```python
from build123d import *

# Parameters (mm, degrees)
SKETCH1_W           = 25.6
SKETCH1_H           = 25.6
BOSS_EXTRUDE1_DEPTH = 15.24
SKETCH2_R           = 2.5
CUT_EXTRUDE1_DEPTH  = 33.426186948
SKETCH3_R           = 1.25
CUT_EXTRUDE2_DEPTH  = 24.663000655
CHAMFER1_SIZE       = 0.5
SKETCH7_R           = 3
CUT_EXTRUDE3_DEPTH  = 24.663000655


with BuildPart() as part:
    # Sketch1 → Boss-Extrude1 (new body)
    with BuildSketch(Plane(origin=(0, 0, 0), x_dir=(1, 0, 0), z_dir=(0, 1, 0))):
        Rectangle(SKETCH1_W, SKETCH1_H)
    extrude(amount=BOSS_EXTRUDE1_DEPTH)

    # Sketch2 → Cut-Extrude1 (cut, through all)
    with BuildSketch(Plane.XY.offset(12.8)):
        with Locations((-8.05, 6.74)):
            Circle(SKETCH2_R)
        with Locations((8.05, 6.74)):
            Circle(SKETCH2_R)
    extrude(amount=-CUT_EXTRUDE1_DEPTH, mode=Mode.SUBTRACT)

    # Sketch3 → Cut-Extrude2 (cut, through all)
    with BuildSketch(Plane(origin=(0, 15.24, 0), x_dir=(1, 0, 0), z_dir=(0, 1, 0))):
        with Locations(Location((0, -8.3, 0), (0, 0, 270))):
            Circle(SKETCH3_R)
    extrude(amount=-CUT_EXTRUDE2_DEPTH, mode=Mode.SUBTRACT)

    # Chamfer1
    chamfer1_edges = [part.edges().sort_by_distance(p)[0] for p in [
        (-10.55, 6.74, -12.8),
        (-10.55, 6.74, 12.8),
        (5.55, 6.74, -12.8),
        (5.55, 6.74, 12.8),
        (0, 0, 7.05),
        (0, 15.24, 7.05),
    ]]
    chamfer(chamfer1_edges, length=CHAMFER1_SIZE)

    # Sketch7 → Cut-Extrude3 (cut, through all)
    with BuildSketch(Plane(origin=(0, 15.24, 0), x_dir=(1, 0, 0), z_dir=(0, 1, 0))):
        with Locations(Location((0, 0, 0), (0, 0, 270))):
            Circle(SKETCH7_R)
    extrude(amount=-CUT_EXTRUDE3_DEPTH, mode=Mode.SUBTRACT)


solid = part.part
```
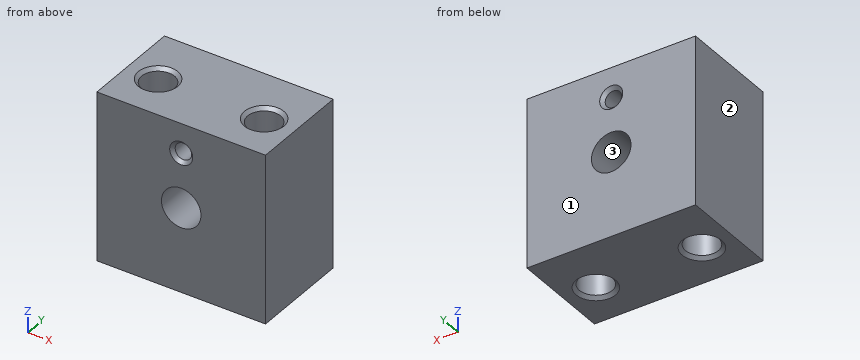
For this review, take the finished solid that the model builds, in its own axes (mm). Face numbers are marked on the shaded views. Give positions to 0.01 mm unless a question says otherwise; leave off trailing zeros. Order: outer loops, then holes, each group sorted by start corner. A loop starts at its lowest first (then second) coordinate and runs counter-clockwise, first axis right, second up.
1) Insertion check: pin 1 (3 mm diameter, centred on x = 0, z = 8.3, fed in from -Y). The pin has a flat end and moves straight along its axis. Give the tip position at first contact, or say it passes through.
2) Wall thickness on line 1 (X direction, y = 8.75, z = 6.5); line 2 (X direction, y = 4.75, z = 7.5); line 3 (Y direction, x = 8.05, z = -2.5): over which ranges is each line inside the solid? List them lowest first.
3) Take a section at B-B (z = 0). Give the boundary of the cut face in (x, y).
4) Take a section at A-A (y = 6.74). Give the boundary of the cut face in (x, z).
5) The part is to be moulded in two halves that separate along X. For the marked faces 1, 2 and 3, say which applies: released by +X, released by -X, zero draft, split by the parting line, or undercut.
6) Take a section at C-C (x = 8.05). Give the boundary of the cut face in (y, z), then the cut area to 3 significant figures.
7) Take a section at D-D (z = -3.5). Give the boundary of the cut face in (x, y), then the cut area to 3 significant figures.
Derived:
1. pin 1: stops at y = 0.25
2. line 1: x = -12.8 to -9.54, -6.56 to 6.56, 9.54 to 12.8
2. line 2: x = -12.8 to -9.56, -6.54 to -0.96, 0.96 to 6.54, 9.56 to 12.8
2. line 3: y = 0 to 4.24, 9.24 to 15.24
3. outline: (-12.8, 0) - (-3, 0) - (-3, 15.24) - (-12.8, 15.24) - close; (3, 0) - (12.8, 0) - (12.8, 15.24) - (3, 15.24) - close; hole circle Ø5 at (-8.05, 6.74); hole circle Ø5 at (8.05, 6.74)
4. outline: (-12.8, -12.8) - (-11.05, -12.8) - (-10.55, -12.3) - (-10.55, 12.3) - (-11.05, 12.8) - (-12.8, 12.8) - close; (-5.55, -12.3) - (-5.05, -12.8) - (5.05, -12.8) - (5.55, -12.3) - (5.55, 12.3) - (5.05, 12.8) - (-5.05, 12.8) - (-5.55, 12.3) - close; (10.55, -12.3) - (11.05, -12.8) - (12.8, -12.8) - (12.8, 12.8) - (11.05, 12.8) - (10.55, 12.3) - close; hole circle Ø6 at (0, 0); hole circle Ø2.5 at (0, 8.3)
5. face 1: zero draft
5. face 2: released by -X
5. face 3: undercut
6. outline: (0, -12.8) - (3.74, -12.8) - (4.24, -12.3) - (4.24, 12.3) - (3.74, 12.8) - (0, 12.8) - close; (9.24, -12.3) - (9.74, -12.8) - (15.24, -12.8) - (15.24, 12.8) - (9.74, 12.8) - (9.24, 12.3) - close
6. area: 262 mm2
7. outline: (-12.8, 0) - (12.8, 0) - (12.8, 15.24) - (-12.8, 15.24) - close; hole circle Ø5 at (-8.05, 6.74); hole circle Ø5 at (8.05, 6.74)
7. area: 351 mm2
